Read the model definition and answer for the solid it produces. Units are mm, in the model's axes. A direction names the side the tool comes from. Give positions to 0.01 mm unless a question says otherwise; leave off trailing zeros. Write each loop counter-clockwise with the first axis right and the second up, starting at its lowest first coordinate (ties: lowest second). Pieces come first, ordered by that corner, then holes. Notation, with made-up numbers: M 0.5,6 L 27.5,6 A14 ccw 27.5,19 Z; hole C -36.75,5 d10. An arc over 180 degrees is marked long. Write each question's results on one line, items separated by ' | '. Start each with the question number.
```python
from build123d import *

# Parameters (mm, degrees)
SKETCH5_W           = 12.880016042
SKETCH5_H           = 15.834691301
CUT_EXTRUDE2_DEPTH  = 7.62
CUT_EXTRUDE6_REACH  = 62
SKETCH11_W          = 3.175
SKETCH11_H          = 3.175
BOSS_EXTRUDE1_DEPTH = 6.35
CUT_EXTRUDE4_DEPTH  = 3.175
SKETCH10_W          = 4
SKETCH10_H          = 0.5
CUT_EXTRUDE5_DEPTH  = 37.349999944
CUT_EXTRUDE7_DEPTH  = 40.64
BOSS_EXTRUDE3_DEPTH = 12.7
SKETCH19_W          = 21.319602533
SKETCH19_H          = 36.10119369
CUT_EXTRUDE10_DEPTH = 13.7
SKETCH21_W          = 9.2375
SKETCH21_H          = 32.92619369
SKETCH21_H_2        = 3.175
BOSS_EXTRUDE4_DEPTH = 3.175
SKETCH15_W          = 6.35
SKETCH15_H          = 3.175
BOSS_EXTRUDE2_DEPTH = 1.5875
SKETCH17_W          = 3.175
SKETCH17_H          = 46.222237063
CUT_EXTRUDE9_DEPTH  = 20
SKETCH22_W          = 28
SKETCH22_H          = 20.25
CUT_EXTRUDE11_DEPTH = 84.59000802
SKETCH23_W          = 1.5875
SKETCH23_H          = 32.92619369
BOSS_EXTRUDE5_DEPTH = 3.175
CUT_EXTRUDE12_DEPTH = 104.974999944


with BuildPart() as part:
    # Sketch2 → Revolve1 (revolve)
    with BuildSketch(Plane(origin=(0, 0, 0), x_dir=(0, 0, -1), z_dir=(1, 0, 0))):
        Polygon((0, -50.8), (-29.999999944, 0), (0, 0), align=None)
    revolve(axis=Axis((0, 0, 0), (0, -1, 0)))

    # Sketch4 → Cut-Revolve1 (revolve, cut)
    with BuildSketch(Plane(origin=(0, 0, 0), x_dir=(0, 0, -1), z_dir=(1, 0, 0))):
        Polygon((0, -45.72), (-24.919999944, 0), (0, 0), align=None)
    revolve(axis=Axis((0, 16.11457811, 0), (0, -1, 0)), mode=Mode.SUBTRACT)

    # Sketch5 → Cut-Extrude2 (cut, symmetric)
    with BuildSketch(Plane(origin=(0, 0, 0), x_dir=(0, 0, -1), z_dir=(1, 0, 0))):
        with Locations((0, -47.812265381)):
            Rectangle(SKETCH5_W, SKETCH5_H)
    extrude(amount=CUT_EXTRUDE2_DEPTH, both=True, mode=Mode.SUBTRACT)

    # Sketch11 → Cut-Extrude6 (cut, up to next)
    with BuildSketch(Plane.XY.offset(29.999999944), mode=Mode.PRIVATE) as cut_extrude6_sk1:
        with Locations((4.7625, -1.5875)):
            Rectangle(SKETCH11_W, SKETCH11_H)
    cut_extrude6_tool1 = extrude(cut_extrude6_sk1.sketch, amount=-CUT_EXTRUDE6_REACH, mode=Mode.PRIVATE) & part.part
    add(cut_extrude6_tool1.solids().sort_by_distance((4.7625, -1.5875, 30))[0], mode=Mode.SUBTRACT)
    # Sketch11 → Cut-Extrude6 (cut, up to next)
    with BuildSketch(Plane.XY.offset(29.999999944), mode=Mode.PRIVATE) as cut_extrude6_sk2:
        with Locations((-4.7625, -1.5875)):
            Rectangle(SKETCH11_W, SKETCH11_H)
    cut_extrude6_tool2 = extrude(cut_extrude6_sk2.sketch, amount=-CUT_EXTRUDE6_REACH, mode=Mode.PRIVATE) & part.part
    add(cut_extrude6_tool2.solids().sort_by_distance((-4.7625, -1.5875, 30))[0], mode=Mode.SUBTRACT)

    # Sketch6 → Boss-Extrude1 (add, symmetric)
    with BuildSketch(Plane(origin=(0, 0, 0), x_dir=(0, 0, -1), z_dir=(1, 0, 0))):
        with BuildLine():
            Line((0, -39.89491973), (-7.374618631, -39.89491973))
            Line((-7.374618631, -39.89491973), (21.419811292, -88.653487823))
            ThreePointArc((21.419811292, -88.653487823), (33.996187642, -103.472377364), (50.8, -113.239496671))
            ThreePointArc((50.8, -113.239496671), (60.639246777, -115.932696949), (70.8, -116.84))
            Line((70.8, -116.84), (73.975, -116.84))
            Line((73.975, -116.84), (73.975, -108.9025))
            Line((73.975, -108.9025), (70.8, -108.9025))
            Line((70.8, -108.9025), (70.8, -110.49))
            ThreePointArc((70.8, -110.49), (45.518672683, -103.782529931), (26.887551662, -85.424507296))
            Line((26.887551662, -85.424507296), (0, -39.89491973))
        make_face()
        Polygon((-30.934610553, 0), (-7.374618631, -39.89491973), (0, -39.89491973), (-23.559991923, 0), align=None)
    extrude(amount=BOSS_EXTRUDE1_DEPTH, both=True)

    # Sketch7 → Cut-Extrude4 (cut)
    with BuildSketch(Plane(origin=(0, 0, 0), x_dir=(0, 0, -1), z_dir=(1, 0, 0))):
        with BuildLine():
            Line((-3.175, -39.89491973), (24.533521366, -86.814682665))
            ThreePointArc((24.533521366, -86.814682665), (41.129063901, -104.288765008), (63.693035948, -112.75178759))
            ThreePointArc((63.693035948, -112.75178759), (67.245408265, -113.217029966), (70.8, -113.665))
            Line((70.8, -113.665), (70.8, -110.49))
            ThreePointArc((70.8, -110.49), (54.803942003, -107.916398221), (40.422357136, -100.455345061))
            ThreePointArc((40.422357136, -100.455345061), (32.902296459, -93.617671422), (26.887551662, -85.424507296))
            Line((26.887551662, -85.424507296), (-23.559991923, 0))
            Line((-23.559991923, 0), (-26.734991923, 0))
            Line((-26.734991923, 0), (-3.175, -39.89491973))
        make_face()
    cut_extrude4 = extrude(amount=-CUT_EXTRUDE4_DEPTH, mode=Mode.SUBTRACT)

    # Mirror1: Cut-Extrude4 across plane
    add(cut_extrude4.mirror(Plane(origin=(0, 0, 0), x_dir=(0, 0, 1), z_dir=(1, 0, 0))), mode=Mode.SUBTRACT)

    # Sketch9 → Cut-Revolve2 (revolve, cut)
    with BuildSketch(Plane(origin=(0, 0, 0), x_dir=(0, 0, -1), z_dir=(1, 0, 0))):
        Polygon((0, 0), (-24.9199908, 0), (-0.536470716, -39.89491973), (0, -39.89491973), align=None)
    revolve(axis=Axis((0, 16.11457811, 0), (0, -1, 0)), mode=Mode.SUBTRACT)

    # Sketch10 → Cut-Extrude5 (cut, through all)
    with BuildSketch(Plane.ZY.offset(6.35)):
        with BuildLine():
            Line((-66.8, -113.665), (-66.8, -110.332889222))
            ThreePointArc((-66.8, -110.332889222), (-68.798457857, -110.450707168), (-70.8, -110.49))
            Line((-70.8, -110.49), (-70.8, -113.665))
            Line((-70.8, -113.665), (-66.8, -113.665))
        make_face()
        with Locations((-68.8, -113.915)):
            Rectangle(SKETCH10_W, SKETCH10_H)
    extrude(amount=-CUT_EXTRUDE5_DEPTH, mode=Mode.SUBTRACT)

    # Sketch12 → Cut-Extrude7 (cut, symmetric)
    with BuildSketch(Plane.ZY):
        Polygon((30, 0), (-61.025869449, 0), (-61.025869449, -39.89491973), (-6.440008021, -39.89491973), (6.44000802, -39.89491973), (27.945214206, -3.175), align=None)
    extrude(amount=CUT_EXTRUDE7_DEPTH, both=True, mode=Mode.SUBTRACT)

    # Sketch18 → Boss-Extrude3 (add)
    with BuildSketch(Plane.ZY.offset(6.35)):
        with BuildLine():
            Line((6.44000802, -39.89491973), (6.44000802, 0))
            Line((6.44000802, 0), (9.61500802, 0))
            Line((9.61500802, 0), (9.61500802, -34.473639686))
            Line((9.61500802, -34.473639686), (9.61500802, -36.10119369))
            ThreePointArc((9.61500802, -36.10119369), (8.57844205, -39.89491973), (5.756782033, -42.634456374))
            Line((5.756782033, -42.634456374), (6.44000802, -41.477527034))
            Line((6.44000802, -41.477527034), (6.44000802, -39.89491973))
        make_face()
    extrude(amount=-BOSS_EXTRUDE3_DEPTH)

    # Sketch19 → Cut-Extrude10 (cut, through all)
    with BuildSketch(Plane.ZY.offset(6.35)):
        with Locations((20.274809287, -18.050596845)):
            Rectangle(SKETCH19_W, SKETCH19_H)
    extrude(amount=-CUT_EXTRUDE10_DEPTH, mode=Mode.SUBTRACT)

    # Sketch21 → Boss-Extrude4 (add)
    with BuildSketch(Plane.XY.offset(9.61500802)):
        with Locations((-10.96875, -19.638096845)):
            Rectangle(SKETCH21_W, SKETCH21_H)
        with Locations((10.96875, -19.638096845)):
            Rectangle(SKETCH21_W, SKETCH21_H)
        with Locations((10.96875, -1.5875)):
            Rectangle(SKETCH21_W, SKETCH21_H_2)
        with Locations((-10.96875, -1.5875)):
            Rectangle(SKETCH21_W, SKETCH21_H_2)
    extrude(amount=-BOSS_EXTRUDE4_DEPTH)

    # Sketch15 → Boss-Extrude2 (add, symmetric)
    with BuildSketch(Plane.ZY.offset(15.5875)):
        with Locations((6.44000802, -1.5875)):
            Rectangle(SKETCH15_W, SKETCH15_H)
    boss_extrude2 = extrude(amount=BOSS_EXTRUDE2_DEPTH, both=True)

    # Mirror2: Boss-Extrude2 across plane
    add(boss_extrude2.mirror(Plane(origin=(0, 0, 0), x_dir=(0, 0, 1), z_dir=(1, 0, 0))))

    # Sketch17 → Cut-Extrude9 (cut)
    with BuildSketch(Plane(origin=(0, 0, -73.975), x_dir=(-1, 0, 0), z_dir=(0, 0, -1))):
        with Locations((-4.7625, -93.728881469)):
            Rectangle(SKETCH17_W, SKETCH17_H)
        with Locations((4.7625, -93.728881469)):
            Rectangle(SKETCH17_W, SKETCH17_H)
    extrude(amount=-CUT_EXTRUDE9_DEPTH, mode=Mode.SUBTRACT)

    # Sketch22 → Cut-Extrude11 (cut, through all)
    with BuildSketch(Plane.XY.offset(9.61500802)):
        with Locations((0, -10.125)):
            Rectangle(SKETCH22_W, SKETCH22_H)
    extrude(amount=-CUT_EXTRUDE11_DEPTH, mode=Mode.SUBTRACT)

    # Sketch23 → Boss-Extrude5 (add)
    with BuildSketch(Plane.XY.offset(9.61500802)):
        with Locations((-16.38125, -19.638096845)):
            Rectangle(SKETCH23_W, SKETCH23_H)
        with Locations((16.38125, -19.638096845)):
            Rectangle(SKETCH23_W, SKETCH23_H)
    extrude(amount=-BOSS_EXTRUDE5_DEPTH)

    # Sketch24 → Cut-Extrude12 (cut, through all)
    with BuildSketch(Plane.XY.offset(29.999999944)):
        Polygon((-17.175, -36.10119369), (-8.68039741, -36.10119369), (-17.175, -21.71699995), align=None)
        Polygon((17.175, -21.71699995), (17.175, -36.10119369), (8.68039741, -36.10119369), align=None)
    extrude(amount=-CUT_EXTRUDE12_DEPTH, mode=Mode.SUBTRACT)


solid = part.part
```
Item 1: Section A-A, the plane y = -19 is taken. Determine the outline of the cut face in (x, z) (3 decimals).
Item 2: Section D-D, the plane y = -96 is taken. Determine the outline of the cut face in (x, z) (3 decimals).
Item 3: Straight lines are drawn through the part: line 1 (Y direction, x = -1.5, z = -70.5) (3 decimals); line 2 (Z direction, x = -13.5, y = -25.5) (3 decimals); line 3 (Y direction, x = 4.5, z = 2). For each, find the intervals that lie inside material, in ascending order.
Item 4: For faces 1 (the cylindrical face through (0.044, -104.1, -40.846)), 2 (the flat face through (16, -3.175, 5)), 3 (the flat face through (14, -10, 8)), 4 (the flat face through (0, -108.902, -72)), determine the directions among +Z, -Z, +X, -X, +Y, -Y from which every point of the face is accessible in a straight line to the end or side of a thin tool.
Item 5: Determine the mould class of faces 5 (the flat face through (16, 0, 6)), 6 (the flat face through (0, -20.25, 8)), 7 (the flat face through (12.87, -29.01, 8.05)) for opening direction X: +X half, -X half, draft (parallel to the pull), parting line (faces both ways), or undercut.
Item 6: Given P1, Ø1, axis at x = 4.5, z = 8, coming from the +Y side; P2, Ø1.9, axis at x = 3, z = 2, coming from the +Y side; P3, Ø2.5, axis at x = 5.5, y = -110, coming from the -Z side (3 decimals), each flat-ended and moving along its own axis, determine where each tip first touches the part or whether it passes through.
Item 7: Section C-C, the plane z = -38 is taken. Determine the outline of the cut face in (x, y) (3 decimals), then the cut area to 3 significant figures.
Worked out:
1) outline: M -17.175,6.44 L -14,6.44 L -14,9.615 L -17.175,9.615 Z; M 14,6.44 L 17.175,6.44 L 17.175,9.615 L 14,9.615 Z
2) outline: M -6.35,-35.192 L -3.175,-35.192 L -3.175,-31.376 L 3.175,-31.376 L 3.175,-35.192 L 6.35,-35.192 L 6.35,-26.574 L -6.35,-26.574 Z
3) line 1: y = -116.839 to -114.165 | line 2: z = 6.44 to 9.615 | line 3: y = -49 to -39.89
4) face 1: +Y | face 2: -Z, +X, -X, -Y | face 3: +Z, -Z, +Y | face 4: -Z, +X, -X, +Y
5) face 5: draft | face 6: undercut | face 7: +X half
6) P1: stops at y = -20.25 | P2: stops at y = -39.89 | P3: stops at z = -53.975
7) outline: M -6.35,-106.534 L 6.35,-106.534 L 6.35,-98.543 L 3.175,-98.543 L 3.175,-102.051 L -3.175,-102.051 L -3.175,-98.543 L -6.35,-98.543 Z | area: 79.2 mm²
